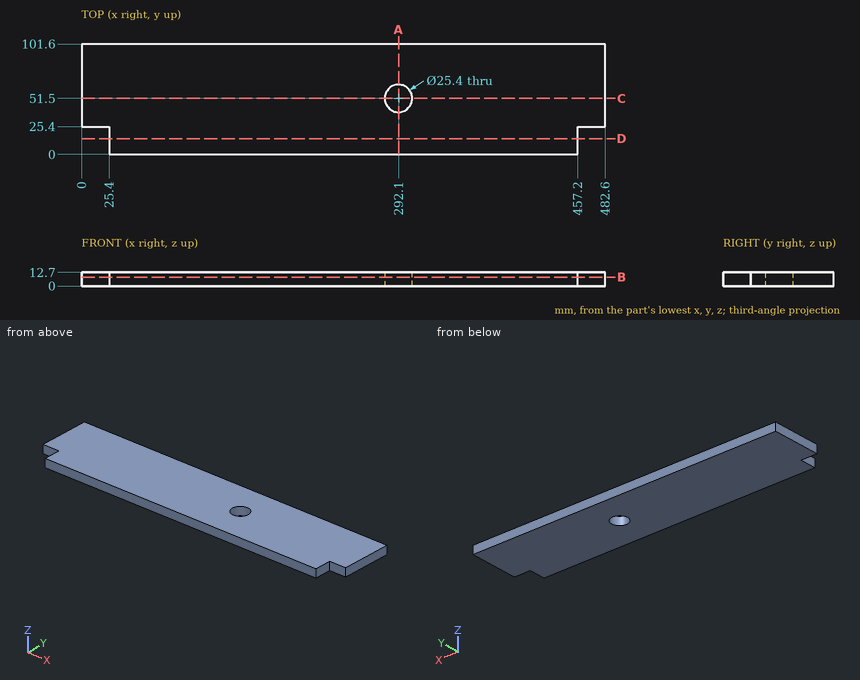
Here's the drawing with two shaded views (mm, measured from the low corner). I have some questions. Give positions to 0.01 mm unless a question says otherwise; leave off trailing zeros. Order: outer loops, then holes, each group sorted by start corner. A loop starts at its lowest first (then second) coordinate and runs counter-clockwise, first axis right, second up. Notation, with made-up numbers: (89.5, 51.25) - (143.5, 51.25) arc R22 ccw to (143.5, 83.25) - close; hole circle Ø1 at (57.25, -32.5). An arc over 180 degrees is marked (long way). Write each question's results on one line, items separated by ' | '.
1) I'm going to push flat-ended pins straight in: pin 1 Ø4 at (y, z) = (7.5, 8) entering from -X; pin 2 Ø6.5 at (y, z) = (9, 9) entering from +X; pin 3 Ø6.5 at (x, z) = (467.5, 5.5) entering from -Y. Where does each tip first touch, or does it pass through?
Final values:
pin 1: stops at x = 25.4 | pin 2: stops at x = 457.2 | pin 3: stops at y = 25.4
2) Suppose I cut it at A-A, the plane x = 292.1. Write out the boundary of the cut face in (y, z), then the cut area to 3 significant figures.
Final values:
outline: (0, 0) - (38.8, 0) - (38.8, 12.7) - (0, 12.7) - close; (64.2, 0) - (101.6, 0) - (101.6, 12.7) - (64.2, 12.7) - close | area: 968 mm^2
3) Suppose I cut it at B-B, the plane z = 8.25. Write out the boundary of the cut face in (x, y).
Final values:
outline: (0, 25.4) - (25.4, 25.4) - (25.4, 0) - (457.2, 0) - (457.2, 25.4) - (482.6, 25.4) - (482.6, 101.6) - (0, 101.6) - close; hole circle Ø25.4 at (292.1, 51.5)
4) Suppose I cut it at C-C, the plane y = 51.5. Write out the boundary of the cut face in (x, z).
Final values:
outline: (0, 0) - (279.4, 0) - (279.4, 12.7) - (0, 12.7) - close; (304.8, 0) - (482.6, 0) - (482.6, 12.7) - (304.8, 12.7) - close
5) Please list where these lines run through material, in increasing order: line 1 along Y through (x, z) = (292.1, 6.5); line 2 along X through (y, z) = (58, 8); line 3 along X through (y, z) = (60.5, 3.75). Write a range as [from, to].
Final values:
line 1: y = [0, 38.8], [64.2, 101.6] | line 2: x = [0, 281.19], [303.01, 482.6] | line 3: x = [0, 283.14], [301.06, 482.6]
6) Suppose I cut it at D-D, the plane y = 14.5. Write out the boundary of the cut face in (x, z), then the cut area to 3 significant figures.
Final values:
outline: (25.4, 0) - (457.2, 0) - (457.2, 12.7) - (25.4, 12.7) - close | area: 5,480 mm^2
